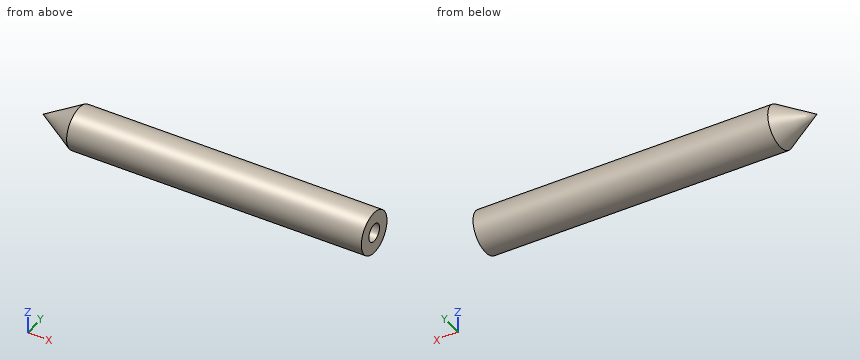
Autodesk Inventor part; units mm, degrees
ref_plane "YZ Plane" through (0, 0, 0) normal (1, 0, 0) x (0, 1, 0)
ref_plane "XZ Plane" through (0, 0, 0) normal (0, 1, 0) x (-1, 0, 0)
ref_plane "XY Plane" through (0, 0, 0) normal (0, 0, 1) x (1, 0, 0)
sketch "Sketch1" plane through (0, 0, 0) normal (1, 0, 0) x (0, 1, 0)
  circle A0 centre (0, 0) radius 4.7625
  dimension "d0" = 9.525
extrude "Extrusion1" add sketch "Sketch1" along normal mid plane 74.93
sketch "Sketch2" plane through (0, 0, 0) normal (0, 1, 0) x (-1, 0, 0)
  line L0 (37.465, -4.7625) -> (37.465, 4.7625)
  line L1 (37.465, 0) -> (29.2161, -4.7625)
  line L2 (37.465, -4.7625) -> (-37.465, -4.7625)
  line L3 (37.465, -4.7625) -> (37.465, 0)
  line L4 (50.2285, 0) -> (-50.2285, 0)
  point P0 (0, 0)
  dimension "d3" = 60
  dimension "d5" = 8.2489
revolve "Revolution1" cut sketch "Sketch2" angle 360 about axis through (-10, 0, 0) along (1, 0, 0)
sketch "Sketch3" plane through (37.465, 0, 0) normal (1, 0, 0) x (0, 0, -1)
  point P0 (0, 0)
  point P1 (0, 0)
hole "Hole1" at (37.465, 0, 0) direction (-1, 0, 0) diameter 3.9624 depth 12.7 tip angle 118
equation "\"d0\" = diam"
equation "\"d1\" = length"
equation "\"diam\" = 9.525"
equation "\"nosePiece_drivenDimesion\" = 8.255"
equation "\"spacerFromOuterTube\" = 3.175"
properties part number "outerTubeStopPost" material "Steel"
Model file for the job. Use its own axes, mm. Give positions to 0.01 mm unless a question says otherwise; leave off trailing zeros. Loops run counter-clockwise (first coordinate to the right, second up) from the corner with the lowest first, then second, coordinate; pieces in that order, holes last. Notation, with made-up numbers: (47, -40) - (96, -40) arc R27 cw to (96, -3) - close; hole circle Ø2 at (83, 66.5). An arc over 180 degrees is marked (long way). One line per item, written item: value. Start each with the question number.
1. Pin check, flat tips, straight feed: pin 1 (1 mm diameter, centred on y = 1.5, z = -1.5, fed in from -X); pin 2 (3 mm diameter, centred on x = -10.5, y = -1, fed in from -Z); pin 3 (1.5 mm diameter, centred on x = -16.5, y = -1.5, fed in from -Z); pin 4 (3 mm diameter, centred on y = 0, z = 0, fed in from +X). Stop position of each tip, or through.
2. Slice it at A-A (x = 30.5). List the corners of the cut face in (y, z) (1 decimal), plus the area to 3 significant figures.
3. Probe L1, parallel to Z at x = 29.75, y = 0; L2, parallel to X at y = -1, z = -1. List the from-to ranges inside material, lowest first. Write a range as from..to.
4. Slice it at B-B (x = 0). List the corners of the cut face in (y, z) (1 decimal), plus the area to 3 significant figures.
Solution:
1. pin 1: stops at x = -34.66
1. pin 2: stops at z = -4.76
1. pin 3: stops at z = -4.7
1. pin 4: stops at x = 24.48
2. outline: circle Ø9.5 at (0, 0); hole circle Ø4 at (0, 0)
2. area: 58.9 mm^2
3. L1: z = -4.76..-1.98, 1.98..4.76
3. L2: x = -35.02..24.42
4. outline: circle Ø9.5 at (0, 0)
4. area: 71.3 mm^2
